```python
from build123d import *

# Parameters (mm, degrees)
SKETCH1_R           = 1.7
BOSS_EXTRUDE1_DEPTH = 12.5
FILLET4_R           = 5
FILLET5_R           = 5
FILLET6_R           = 5
FILLET7_R           = 20
SKETCH2_R           = 1.745
CUT_EXTRUDE1_DEPTH  = 10
CUT_EXTRUDE2_DEPTH  = 35
FILLET8_R           = 5
FILLET9_R           = 5


with BuildPart() as part:
    # Sketch1 → Boss-Extrude1 (new body)
    with BuildSketch(Plane.XY):
        with BuildLine():
            Line((-56.849444808, -8.625), (-54.713862361, -22.701136402))
            Line((-54.713862361, -22.701136402), (-14.786422414, -154.047675233))
            Line((-14.786422414, -154.047675233), (15.213577586, -154.047675233))
            Line((15.213577586, -154.047675233), (37.488789117, -55.269230384))
            Line((37.488789117, -55.269230384), (30.258636425, -33.307880775))
            ThreePointArc((30.258636425, -33.307880775), (-9.886965016, -43.90043192), (-41.615847066, -17.120784823))
            ThreePointArc((-41.615847066, -17.120784823), (-47.779287866, -10.266909246), (-56.849444808, -8.625))
        make_face()
        with Locations((0, -52)):
            Circle(SKETCH1_R, mode=Mode.SUBTRACT)
        with Locations((-26, -45.033320997)):
            Circle(SKETCH1_R, mode=Mode.SUBTRACT)
        with Locations((-45.033320997, -26)):
            Circle(SKETCH1_R, mode=Mode.SUBTRACT)
        with Locations((26, -45.033320997)):
            Circle(SKETCH1_R, mode=Mode.SUBTRACT)
    extrude(amount=BOSS_EXTRUDE1_DEPTH)

    # Fillet4
    fillet4_edges = [part.edges().sort_by_distance(p)[0] for p in [
        (-56.849444808, -8.625, 6.25),
    ]]
    fillet(fillet4_edges, radius=FILLET4_R)

    # Fillet5
    fillet5_edges = [part.edges().sort_by_distance(p)[0] for p in [
        (-54.713862361, -22.701136402, 6.25),
    ]]
    fillet(fillet5_edges, radius=FILLET5_R)

    # Fillet6
    fillet6_edges = [part.edges().sort_by_distance(p)[0] for p in [
        (30.258636425, -33.307880775, 6.25),
    ]]
    fillet(fillet6_edges, radius=FILLET6_R)

    # Fillet7
    fillet7_edges = [part.edges().sort_by_distance(p)[0] for p in [
        (37.488789117, -55.269230384, 6.25),
    ]]
    fillet(fillet7_edges, radius=FILLET7_R)

    # Sketch2 → Cut-Extrude1 (cut)
    with BuildSketch(Plane(origin=(0, -154.047675233, 0), x_dir=(-1, 0, 0), z_dir=(0, -1, 0))):
        with Locations(Location((-0.213577586, -6.25, 0), (0, 0, 90))):
            Circle(SKETCH2_R)
    extrude(amount=-CUT_EXTRUDE1_DEPTH, mode=Mode.SUBTRACT)

    # Sketch3 → Cut-Extrude2 (cut)
    with BuildSketch(Plane(origin=(0, 0, 0), x_dir=(-1, 0, 0), z_dir=(0, 0, -1))):
        with BuildLine():
            Line((-19.010121999, -64.01448337), (-2.601927454, -139.726581059))
            Line((-2.601927454, -139.726581059), (24.588794936, -61.670455578))
            ThreePointArc((24.588794936, -61.670455578), (3.57566323, -77.468147247), (-19.010121999, -64.01448337))
        make_face()
    extrude(amount=-CUT_EXTRUDE2_DEPTH, mode=Mode.SUBTRACT)

    # Fillet8
    fillet8_edges = [part.edges().sort_by_distance(p)[0] for p in [
        (2.601927454, -139.726581059, 6.25),
    ]]
    fillet(fillet8_edges, radius=FILLET8_R)

    # Fillet9
    fillet9_edges = [part.edges().sort_by_distance(p)[0] for p in [
        (19.010121999, -64.01448337, 6.25),
    ]]
    fillet(fillet9_edges, radius=FILLET9_R)
    fillet9_2_edges = [part.edges().sort_by_distance(p)[0] for p in [
        (-24.588794936, -61.670455578, 6.25),
    ]]
    fillet(fillet9_2_edges, radius=FILLET9_R)


solid = part.part
```
CAD build for the part. Positions are in the model's coordinates, mm. A direction names the side the tool comes from. Round coordinates to 2 decimals unless told otherwise and drop trailing zeros. Write each loop counter-clockwise with the first axis right and the second up, starting at its lowest first coordinate (ties: lowest second). Pieces come first, ordered by that corner, then holes. Notation, with made-up numbers: (31, 10) - (49, 10) arc R20 cw to (49, 36) - close; hole circle Ø7 at (-14.5, 60). An arc over 180 degrees is marked (long way). Return JSON: item names as keys, results as strings. Group by question number.
Item 1: 3-axis set-ups, long thin cutter, end or side, ignore diameter. For faces 1 (the face through (0, -144.048, 6)), 2 (the face through (-1.342, -77.482, 6.162)), 3 (the face through (29.3, -36.86, 6.34)): which of +Z, -Z, +X, -X, +Y, -Y reach the whole face in a straight line?
Item 2: Probe probe 1 along Y at (x, z) = (0, 5); probe 2 along Y at (x, z) = (3.5, 1.5); probe 3 along X at (y, z) = (-98, 11). List the from-to ranges inside material, lowest first.
Item 3: Band-saw the part on A-A on x = -26. List the corners of the cut face in (y, z), plus the area to 3 significant figures.
Item 4: Band-saw the part on D-D on x = 31. List the corners of the cut face in (y, z), plus the area to 3 significant figures.
Item 5: Mould opens along X. For faces 4 (the face through (34.14, -45.1, 6.16)), 5 (the face through (-43.41, -25.49, 6.16)), 6 (the face through (-54.021, -10.337, 6.338)), 7 (the face through (-21, -81, 0)) say: +X half, -X half, draft (parallel to the pull), parting line (faces both ways), or undercut.
Item 6: Band-saw the part on B-B on y = -117. List the corners of the cut face in (x, z), plus the area to 3 significant figures.
Item 7: Flat gauge pins, fed straight in: pin 1 Ø2 at (x, z) = (0.21, 6.25) entering from +Y; pin 2 Ø3 at (x, z) = (-3.5, 8.5) entering from +Y. Where does each tip first touch, or does it go through?
Item 8: Band-saw the part on C-C on z = 10.25. List the corners of the cut face in (x, y).
Resolved:
{
 "1": {"face 1": "-Y", "face 2": "+Z, -Z", "face 3": "+Z, -Z, +Y"},
 "2": {"probe 1": "y = -144.05 to -126.08, -77.39 to -53.7, -50.3 to -45", "probe 2": "y = -154.05 to -125.88, -76.78 to -44.86", "probe 3": "x = -31.82 to -11.93, 11.64 to 27.85"},
 "3": {"outline": "(-117.16, 0) - (-46.73, 0) - (-46.73, 12.5) - (-117.16, 12.5) - close; (-43.33, 0) - (-36.73, 0) - (-36.73, 12.5) - (-43.33, 12.5) - close", "area": "963 mm²"},
 "4": {"outline": "(-84.04, 0) - (-37.83, 0) - (-37.83, 12.5) - (-84.04, 12.5) - close", "area": "578 mm²"},
 "5": {"face 4": "+X half", "face 5": "undercut", "face 6": "parting line", "face 7": "draft"},
 "6": {"outline": "(-26.05, 0) - (-5.31, 0) - (-5.31, 12.5) - (-26.05, 12.5) - close; (7.53, 0) - (23.57, 0) - (23.57, 12.5) - (7.53, 12.5) - close", "area": "460 mm²"},
 "7": {"pin 1": "stops at y = -44.98", "pin 2": "stops at y = -44.72"},
 "8": {"outline": "(-55.88, -15.02) - (-54.77, -22.34) arc R5 ccw to (-54.61, -23.05) - (-14.79, -154.05) - (15.21, -154.05) - (36.27, -60.67) arc R20 ccw to (35.76, -50.01) - (32.48, -40.04) arc R5 ccw to (24.95, -37.45) arc R45 cw to (-41.62, -17.12) arc R14.24 ccw to (-48.89, -9.71) arc R5 ccw to start; hole circle Ø3.4 at (-45.03, -26); hole circle Ø3.4 at (-26, -45.03); hole (-17.44, -82.18) - (-3.24, -122.95) arc R5 ccw to (6.37, -122.36) - (15.44, -80.51) arc R5 ccw to (8.3, -74.98) arc R23.59 cw to (-10.9, -75.88) arc R5 ccw to start; hole circle Ø3.4 at (0, -52); hole circle Ø3.4 at (26, -45.03)"}
}
